Could you check a few things on this model? Use its own coordinates, in mm. Face numbers are marked on the shaded views. Give positions to 0.01 mm unless a question says otherwise; leave off trailing zeros. Loops run counter-clockwise (first coordinate to the right, second up) from the corner with the lowest first, then second, coordinate; pieces in that order, holes last. Notation, with made-up numbers: (0.5, 45) -> (8.5, 45) arc R22 ccw to (8.5, 72) -> close; hole circle Ø9 at (87.5, 65.5). An arc over 180 degrees is marked (long way). Write each question's results on one line, items separated by ' | '. Start each with the question number.
Q1. If we section it at C-C, the plane z = 27: List the corners of the cut face in (x, y) for me.
Q2. If I drill on line 1 along Y through (x, z) = (0, 12); line 2 along Y through (x, z) = (-7, 22); line 3 along Y through (x, z) = (24, 28), over which ranges is the centre line in solid material (lowest first)?
Q3. Will these pins go through, and if not, where does the flat tip stop? P1, Ø1.5, axis at x = 1, z = 5.5, coming from the -Y side; P2, Ø1.5, axis at x = -7.5, z = 13, coming from the +Y side; P3, Ø8, axis at y = -17.5, z = 20.5, coming from the +X side.
Q4. We'd pull the mould along Y, two halves only. Please class the marked faces 1, 2 and 3: released by +Y, released by -Y, zero draft, split by the parting line, or undercut.
Q5. If we section it at A-A, the plane y = 0: List the corners of the cut face in (x, z) for me, plus the area to 3 significant figures.
from build123d import *

# Parameters (mm, degrees)
SKETCH1_R           = 35
BOSS_EXTRUDE1_DEPTH = 42
FILLET1_R           = 3
SKETCH2_R           = 11
CUT_EXTRUDE1_DEPTH  = 65.915329522


with BuildPart() as part:
    # Sketch1 → Boss-Extrude1 (new body)
    with BuildSketch(Plane.XY):
        with Locations(Location((0, 0, 0), (0, 0, 180))):
            Circle(SKETCH1_R)
    extrude(amount=BOSS_EXTRUDE1_DEPTH)

    # Fillet1
    fillet1_edges = [part.edges().sort_by_distance(p)[0] for p in [
        (35, 0, 0),
        (35, 0, 42),
    ]]
    fillet(fillet1_edges, radius=FILLET1_R)

    # Sketch2 → Cut-Extrude1 (cut, through all)
    with BuildSketch(Plane.XY.offset(42)):
        Circle(SKETCH2_R)
    extrude(amount=-CUT_EXTRUDE1_DEPTH, mode=Mode.SUBTRACT)


solid = part.part
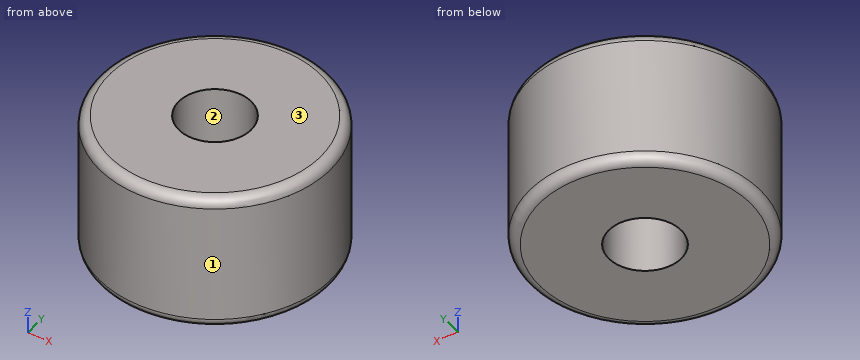
Final values:
1) outline: circle Ø70 at (0, 0); hole circle Ø22 at (0, 0)
2) line 1: y = -35 to -11, 11 to 35 | line 2: y = -34.29 to -8.49, 8.49 to 34.29 | line 3: y = -25.48 to 25.48
3) P1: stops at y = -35 | P2: stops at y = 34.34 | P3: stops at x = 32.29
4) face 1: split by the parting line | face 2: undercut | face 3: zero draft
5) outline: (-35, 3) arc R3 ccw to (-32, 0) -> (-11, 0) -> (-11, 42) -> (-32, 42) arc R3 ccw to (-35, 39) -> close; (11, 0) -> (32, 0) arc R3 ccw to (35, 3) -> (35, 39) arc R3 ccw to (32, 42) -> (11, 42) -> close | area: 2,010 mm²
